Source: CAD feature listing. Evaluate the final solid. Frame: model axes, mm. Face numbers are marked on the shaded views. Coordinates: 2 decimals unless noted, no trailing zeros. Loops run counter-clockwise (first coordinate to the right, second up) from the corner with the lowest first, then second, coordinate; pieces in that order, holes last. Notation, with made-up numbers: (-26.75, -12.5) -> (12.25, -12.5) arc R18 cw to (12.25, 5.5) -> close; hole circle Ø8 at (27, -13). An arc over 180 degrees is marked (long way). Answer as CSV lines item,"result".
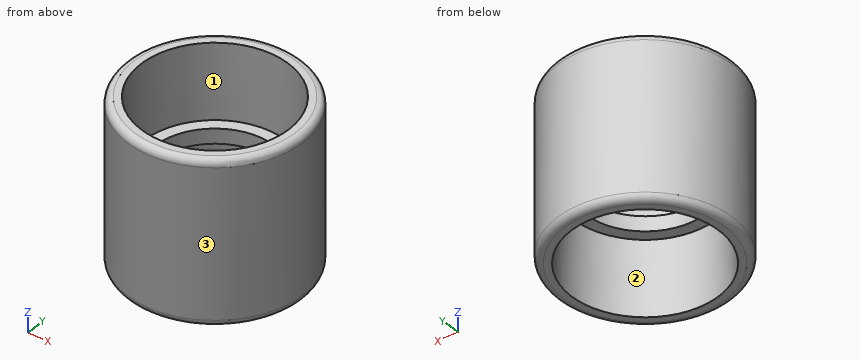
from build123d import *

# Parameters (mm, degrees)
BODYSCH_R  = 9.5
BODY_DEPTH = 8.8
FLOWSCH_R  = 6.5
FLOW_DEPTH = 17.6
FILLET1_R  = 0.75


with BuildPart() as part:
    # BodySch → Body (new, symmetric)
    with BuildSketch(Plane.XY):
        Circle(BODYSCH_R)
    extrude(amount=BODY_DEPTH, both=True)

    # FlowSch → Flow (cut)
    with BuildSketch(Plane.XY.offset(-8.8)):
        Circle(FLOWSCH_R)
    extrude(amount=FLOW_DEPTH, mode=Mode.SUBTRACT)

    # ThreadSch → Thread (revolve, cut)
    with BuildSketch(Plane(origin=(0, 0, 0), x_dir=(0, 0, -1), z_dir=(1, 0, 0))):
        Polygon((-0.8, 0), (-0.8, 7.750919254), (-8.8, 8), (-8.8, 0), align=None)
    thread = revolve(axis=Axis((0, 0, 0), (0, 0, 1)), mode=Mode.SUBTRACT)

    # Fillet1
    fillet1_edges = [part.edges().sort_by_distance(p)[0] for p in [
        (-9.5, 0, -8.8),
        (-9.5, 0, 8.8),
    ]]
    fillet(fillet1_edges, radius=FILLET1_R)

    # Mirror1: Thread across plane
    add(thread.mirror(Plane.XY), mode=Mode.SUBTRACT)


solid = part.part
(1) Cut plane C-C (z = 5.75). Return the cut outline in (x, y).
Computed values:
outline,"circle Ø19 at (0, 0); hole circle Ø15.81 at (0, 0)"
(2) Material intervals for L1, parallel to Y at x = 0, z = -0.05; L2, parallel to Z at x = -2.25, y = 8.5; L3, parallel to X at y = -3.5, z = -6.5, sorted ascending. Write a range as [from, to].
Computed values:
L1,"[-9.5, -6.5], [6.5, 9.5]"
L2,"[-8.8, 8.8]"
L3,"[-8.83, -7.11], [7.11, 8.83]"
(3) Draft query along Y for the marked faces 1, 2 and 3. Return one class per face: released by +Y, released by -Y, zero draft, split by the parting line, or undercut.
Computed values:
face 1,"undercut"
face 2,"undercut"
face 3,"split by the parting line"
(4) Cut plane D-D (z = -4.75). Return the cut outline in (x, y).
Computed values:
outline,"circle Ø19 at (0, 0); hole circle Ø15.75 at (0, 0)"
(5) Pin query (flat end, axial travel): pin 1 Ø1.5 at (y, z) = (-5, -6.5) entering from -X; pin 2 Ø8 at (x, z) = (-5, -5.5) entering from -Y; pin 3 Ø8 at (x, y) = (0, 0) entering from +Z; pin 4 Ø1.5 at (y, z) = (7, 2.5) entering from +X. Return the tip coordinate at first contact, or that it passes through.
Computed values:
pin 1,"x = -8.5"
pin 2,"y = -9.45"
pin 3,"through"
pin 4,"x = 7.15"
(6) Cut plane A-A (x = 0). Return the cut outline in (y, z), then the cut area to 3 significant figures.
Computed values:
outline,"(-9.5, -8.05) arc R0.75 ccw to (-8.75, -8.8) -> (-8, -8.8) -> (-7.75, -0.8) -> (-6.5, -0.8) -> (-6.5, 0.8) -> (-7.75, 0.8) -> (-8, 8.8) -> (-8.75, 8.8) arc R0.75 ccw to (-9.5, 8.05) -> close; (6.5, -0.8) -> (7.75, -0.8) -> (8, -8.8) -> (8.75, -8.8) arc R0.75 ccw to (9.5, -8.05) -> (9.5, 8.05) arc R0.75 ccw to (8.75, 8.8) -> (8, 8.8) -> (7.75, 0.8) -> (6.5, 0.8) -> close"
area,"61.1 mm^2"
